```python
from build123d import *

# Parameters (mm, degrees)
CHAMFER_1_SIZE      = 0.2
CHAMFER_1_SIZE_2    = 0.549495484
FILLET_1_R          = 0.5
CUT_EXTRUDE_1_DEPTH = 1.2


with BuildPart() as part:
    # Sketch1 → Revolve1 (revolve)
    with BuildSketch(Plane.XY, mode=Mode.PRIVATE) as revolve1_sk:
        with BuildLine():
            Line((0, 68.75), (-2.5, 68.75))
            Line((-2.5, 68.75), (-3.1, 67.55))
            Line((-3.1, 67.55), (-6.5, 67.55))
            Line((-6.5, 67.55), (-6.5, 67.8))
            Line((-6.5, 67.8), (-8.625, 67.8))
            Line((-8.625, 67.8), (-9.275, 67.15))
            Line((-9.275, 67.15), (-9.275, 61.45))
            ThreePointArc((-9.275, 61.45), (-8.9, 60.5), (-9.275, 59.55))
            Line((-9.275, 59.55), (-9.275, 2))
            Line((-9.275, 2), (-9.1, 2))
            Line((-9.1, 2), (-9.1, 0))
            Line((-9.1, 0), (-7, 0))
            Line((-7, 0), (-7, 0.25))
            Line((-7, 0.25), (0, 0.25))
            Line((0, 0.25), (0, 68.75))
        make_face()
    revolve(revolve1_sk.sketch.rotate(Axis((0, 93.422769263, 0), (0, -1, 0)), 270), axis=Axis((0, 93.422769263, 0), (0, -1, 0)))

    # Фаска1
    # the kernel refuses this chamfer: 0.549495484, 0.2 mm, written as the material it adds along each edge
    with BuildSketch(Plane(origin=(0, 2, 0), x_dir=(0, 0, 1), z_dir=(1, 0, 0))) as chamfer_1_piece_1_section:
        Polygon((9.1 + CHAMFER_1_SIZE, 0), (9.1, CHAMFER_1_SIZE_2), (9.1, 0), align=None)
    chamfer_1_piece_1 = revolve(axis=Axis((0, 2, 0), (0, -1, 0)), mode=Mode.PRIVATE)
    chamfer_1_piece_1 = chamfer_1_piece_1 & Plane(origin=(0, 1.685840324, 0), x_dir=(0, 0, 1), z_dir=(0, -1, 0)) * Cylinder(9.275, 38, mode=Mode.PRIVATE)
    add(chamfer_1_piece_1)

    # Скругление1
    fillet_1_edges = [part.edges().sort_by_distance(p)[0] for p in [
        (0, 61.45, -9.275),
        (0, 59.55, -9.275),
        (0, 68.75, -2.5),
    ]]
    fillet(fillet_1_edges, radius=FILLET_1_R)

    # Эскиз1 → Вырез-Вытянуть1 (cut)
    with BuildSketch(Plane(origin=(0, 68.75, 0), x_dir=(1, 0, 0), z_dir=(0, 1, 0))):
        with BuildLine():
            Line((-2.830089464, -0.470245053), (-3.050819562, -0.55))
            ThreePointArc((-3.050819562, -0.55), (-3.1, 0), (-3.050819562, 0.55))
            Line((-3.050819562, 0.55), (-2.830089464, 0.470245053))
            ThreePointArc((-2.830089464, 0.470245053), (-2.5, 0), (-2.830089464, -0.470245053))
        make_face()
        with BuildLine():
            Line((2.830089464, 0.470245053), (3.050819562, 0.55))
            ThreePointArc((3.050819562, 0.55), (3.1, 0), (3.050819562, -0.55))
            Line((3.050819562, -0.55), (2.830089464, -0.470245053))
            ThreePointArc((2.830089464, -0.470245053), (2.5, 0), (2.830089464, 0.470245053))
        make_face()
    extrude(amount=-CUT_EXTRUDE_1_DEPTH, mode=Mode.SUBTRACT)


solid = part.part
```
Source: CAD feature listing. Evaluate the final solid. Frame: model axes, mm. A direction names the side the tool comes from. Round coordinates to 2 decimals unless told otherwise and drop trailing zeros. Loops run counter-clockwise (first coordinate to the right, second up) from the corner with the lowest first, then second, coordinate; pieces in that order, holes last.
1. Mould query, pull axis Z, two halves, no side actions, for faces 4 (the flat face through (3, 67.55, 0)), 5 (the cylindrical face through (-2.786, 64.351, 8.847)), 6 (the flat face through (0, 68.75, 0)). Classes: released by +Z, released by -Z, zero draft, split by the parting line, or undercut.
2. Contact query for flat-ended pins moving along their axis: pin 1 (8 mm diameter, centred on x = -5, y = 13.5, fed in from +Z); pin 2 (5 mm diameter, centred on x = 1, z = 6.5, fed in from +Y); pin 3 (4 mm diameter, centred on x = 4, y = 37.5, fed in from +Z); pin 4 (11 mm diameter, centred on x = 2.5, z = 1, fed in from -Y). Output: stop coordinate, or through.
3. Section query A-A on y = 7. Output: boundary loops of the cut face in (x, z) (3 decimals).
4. Access query for faces 1 (the cylindrical face through (5.54, 0.72, -7.22)), 2 (the conical face through (-0.06, 68.31, -2.72)), 3 (the cylindrical face through (-7.82, 30.25, 4.99)). Directions: +Z, -Z, +X, -X, +Y, -Y. A direction counts if a zero-diameter tool reaches every point of the face in a straight line with its end or side. Return the directions, or none.
5. Ray query, L1, parallel to X at y = 0.1, z = 0; L2, parallel to X at y = 67.65, z = 0 (3 decimals); L3, parallel to Y at x = 1.75, z = 3.25. Return the intervals inside material, ascending.
Answers below:
1. face 4: undercut
1. face 5: split by the parting line
1. face 6: zero draft
2. pin 1: stops at z = 9.22
2. pin 2: stops at y = 67.8
2. pin 3: stops at z = 9.06
2. pin 4: stops at y = 0
3. outline: circle Ø18.55 at (0, 0)
4. face 1: -Y
4. face 2: +Y
4. face 3: +Y, -Y
5. L1: x = -9.1 to -7, 7 to 9.1
5. L2: x = -8.775 to -6.5, -2.5 to 2.5, 6.5 to 8.775
5. L3: y = 0.25 to 67.55
